from build123d import *

# Parameters (mm, degrees)
SKETCH1_W           = 50.8
SKETCH1_H           = 76.2
BOSS_EXTRUDE2_DEPTH = 20
SKETCH2_R           = 3.7
BOSS_EXTRUDE3_DEPTH = 2
CHAMFER7_SIZE       = 2.222212054
CHAMFER7_SIZE_2     = 25.4
FILLET6_R           = 2
FILLET7_R           = 2
FILLET8_R           = 2
FILLET9_R           = 2
FILLET10_R          = 2


with BuildPart() as part:
    # Sketch1 → Boss-Extrude2 (new body)
    with BuildSketch(Plane(origin=(0, 0, 0), x_dir=(1, 0, 0), z_dir=(0, 1, 0))):
        Rectangle(SKETCH1_W, SKETCH1_H)
    extrude(amount=BOSS_EXTRUDE2_DEPTH)

    # Sketch2 → Boss-Extrude3 (add)
    with BuildSketch(Plane(origin=(0, 0, -38.1), x_dir=(-1, 0, 0), z_dir=(0, 0, -1))):
        with Locations((-15.4, 10)):
            Circle(SKETCH2_R)
        with Locations((15.4, 10)):
            Circle(SKETCH2_R)
    extrude(amount=BOSS_EXTRUDE3_DEPTH)

    # Chamfer7
    # the kernel refuses this chamfer: 25.4, 2.222212054 mm, written as the material it takes off along each edge
    with BuildSketch(Plane(origin=(-25.4, -66.030705628, -38.1), x_dir=(-0.40120984275090654, 0, 0.9159861691531116), z_dir=(0, 1, 0))) as chamfer7_piece_1_section:
        Polygon((CHAMFER7_SIZE * 0.915986168971, CHAMFER7_SIZE * 0.401209842671), (-CHAMFER7_SIZE_2 * 0.401209842751, CHAMFER7_SIZE_2 * 0.915986169153), (0, 0), align=None)
    chamfer7_piece_1 = extrude(amount=152.061411256, mode=Mode.PRIVATE)
    chamfer7_piece_1 = chamfer7_piece_1 - Plane(origin=(-15.4, 10, -36.375506271), x_dir=(-1, 0, 0), z_dir=(0, 0, 1)) * Cylinder(3.7, 398, mode=Mode.PRIVATE)
    add(chamfer7_piece_1, mode=Mode.SUBTRACT)
    with BuildSketch(Plane(origin=(25.4, -66.030705628, -38.1), x_dir=(0.4012098427509076, 0, 0.9159861691531113), z_dir=(0, 1, 0))) as chamfer7_piece_2_section:
        Polygon((CHAMFER7_SIZE * 0.915986168971, -CHAMFER7_SIZE * 0.401209842671), (-CHAMFER7_SIZE_2 * 0.401209842751, -CHAMFER7_SIZE_2 * 0.915986169153), (0, 0), align=None)
    chamfer7_piece_2 = extrude(amount=152.061411256, mode=Mode.PRIVATE)
    chamfer7_piece_2 = chamfer7_piece_2 - Plane(origin=(15.4, 10, -36.375506337), x_dir=(-1, 0, 0), z_dir=(0, 0, 1)) * Cylinder(3.7, 398, mode=Mode.PRIVATE)
    add(chamfer7_piece_2, mode=Mode.SUBTRACT)

    # Fillet6
    fillet6_edges = [part.edges().sort_by_distance(p)[0] for p in [
        (25.4, 20, 1.111106027),
        (0, 20, 38.1),
        (12.7, 20, -36.988893973),
        (-12.7, 20, -36.988893973),
        (-25.4, 20, 1.111106027),
    ]]
    fillet(fillet6_edges, radius=FILLET6_R)

    # Fillet7
    # the kernel refuses this fillet: 2 mm, written as the material it takes off along each edge
    with BuildSketch(Plane(origin=(23.4, 18, -34.045125598), x_dir=(1, 0, 0), z_dir=(0, 1, 0))) as fillet7_piece_1_section:
        Polygon((0, 0), (FILLET7_R, 0), (FILLET7_R, FILLET7_R * 0.916331174017), (FILLET7_R * 0.0871557427476, FILLET7_R * 0.996194698092), align=None)
    fillet7_piece_1 = extrude(amount=FILLET7_R, mode=Mode.PRIVATE)
    fillet7_piece_1 = fillet7_piece_1 - Plane(origin=(23.4, 18, -34.045125598), x_dir=(-0.73727733681012, 0, 0.6755902076156647), z_dir=(0, 1, 0)) * Sphere(FILLET7_R, mode=Mode.PRIVATE)
    add(fillet7_piece_1, mode=Mode.SUBTRACT)
    with BuildSketch(Plane(origin=(25.4, -4.58165587, -35.877787946), x_dir=(0, 0, 1), z_dir=(0, 1, 0))) as fillet7_piece_2:
        with BuildLine():
            CenterArc((FILLET7_R * 0.916331174017, -FILLET7_R), FILLET7_R, 90, 85)
            Line((-FILLET7_R * 0.0798635240743, -FILLET7_R * 0.912844257252), (0, 0))
            Line((0, 0), (FILLET7_R * 0.916331174017, 0))
        make_face()
    extrude(amount=22.58165587, mode=Mode.SUBTRACT)

    # Fillet8
    # the kernel refuses this fillet: 2 mm, written as the material it takes off along each edge
    with BuildSketch(Plane(origin=(23.4, 18, 36.1), x_dir=(1, 0, 0), z_dir=(0, 0, 1))) as fillet8_piece_1_section:
        Polygon((0, 0), (FILLET8_R, 0), (FILLET8_R, FILLET8_R), (0, FILLET8_R), align=None)
    fillet8_piece_1 = extrude(amount=FILLET8_R, mode=Mode.PRIVATE)
    fillet8_piece_1 = fillet8_piece_1 - Plane(origin=(23.4, 18, 36.1), x_dir=(-0.7071067811865475, -0.7071067811865475, 0), z_dir=(0, 0, 1)) * Sphere(FILLET8_R, mode=Mode.PRIVATE)
    add(fillet8_piece_1, mode=Mode.SUBTRACT)
    with BuildSketch(Plane(origin=(25.4, -5, 38.1), x_dir=(-1, 0, 0), z_dir=(0, 1, 0))) as fillet8_piece_2:
        with BuildLine():
            CenterArc((FILLET8_R, -FILLET8_R), FILLET8_R, 90, 90)
            Line((0, -FILLET8_R), (0, 0))
            Line((0, 0), (FILLET8_R, 0))
        make_face()
    extrude(amount=23, mode=Mode.SUBTRACT)

    # Fillet9
    # the kernel refuses this fillet: 2 mm, written as the material it takes off along each edge
    with BuildSketch(Plane(origin=(-23.4, 18, 36.1), x_dir=(-1, 0, 0), z_dir=(0, 0, 1))) as fillet9_piece_1_section:
        Polygon((0, 0), (FILLET9_R, 0), (FILLET9_R, -FILLET9_R), (0, -FILLET9_R), align=None)
    fillet9_piece_1 = extrude(amount=FILLET9_R, mode=Mode.PRIVATE)
    fillet9_piece_1 = fillet9_piece_1 - Plane(origin=(-23.4, 18, 36.1), x_dir=(0.7071067811865475, -0.7071067811865475, 0), z_dir=(0, 0, 1)) * Sphere(FILLET9_R, mode=Mode.PRIVATE)
    add(fillet9_piece_1, mode=Mode.SUBTRACT)
    with BuildSketch(Plane(origin=(-25.4, -5, 38.1), x_dir=(1, 0, 0), z_dir=(0, 1, 0))) as fillet9_piece_2:
        with BuildLine():
            CenterArc((FILLET9_R, FILLET9_R), FILLET9_R, 180, 90)
            Line((0, FILLET9_R), (0, 0))
            Line((0, 0), (FILLET9_R, 0))
        make_face()
    extrude(amount=23, mode=Mode.SUBTRACT)

    # Fillet10
    # the kernel refuses this fillet: 2 mm, written as the material it takes off along each edge
    with BuildSketch(Plane(origin=(-23.4, 18, -34.045125598), x_dir=(-1, 0, 0), z_dir=(0, 1, 0))) as fillet10_piece_1_section:
        Polygon((0, 0), (FILLET10_R, 0), (FILLET10_R, -FILLET10_R * 0.916331174017), (FILLET10_R * 0.0871557427476, -FILLET10_R * 0.996194698092), align=None)
    fillet10_piece_1 = extrude(amount=FILLET10_R, mode=Mode.PRIVATE)
    fillet10_piece_1 = fillet10_piece_1 - Plane(origin=(-23.4, 18, -34.045125598), x_dir=(0.73727733681012, 0, 0.6755902076156647), z_dir=(0, 1, 0)) * Sphere(FILLET10_R, mode=Mode.PRIVATE)
    add(fillet10_piece_1, mode=Mode.SUBTRACT)
    with BuildSketch(Plane(origin=(-25.4, -4.58165587, -35.877787946), x_dir=(0, 0, 1), z_dir=(0, 1, 0))) as fillet10_piece_2:
        with BuildLine():
            CenterArc((FILLET10_R * 0.916331174017, FILLET10_R), FILLET10_R, 185, 85)
            Line((-FILLET10_R * 0.0798635240743, FILLET10_R * 0.912844257252), (0, 0))
            Line((0, 0), (FILLET10_R * 0.916331174017, 0))
        make_face()
    extrude(amount=22.58165587, mode=Mode.SUBTRACT)


solid = part.part
CAD build for the part. Positions are in the model's coordinates, mm. A direction names the side the tool comes from. Round coordinates to 2 decimals unless told otherwise and drop trailing zeros. Write each loop counter-clockwise with the first axis right and the second up, starting at its lowest first coordinate (ties: lowest second). Pieces come first, ordered by that corner, then holes. Notation, with made-up numbers: (25.25, 73) -> (30.25, 73) arc R16 ccw to (30.25, 103) -> close; hole circle Ø9 at (80, 42.5). An arc over 180 degrees is marked (long way). Answer as a JSON object with one key per item and string values.
(1) Band-saw the part on B-B, the plane y = 12. List the corners of the cut face in (x, z).
Reported:
{"outline": "(-25.4, -34.05) arc R2 ccw to (-23.57, -36.04) -> (-18.51, -36.48) -> (-18.51, -40.1) -> (-12.29, -40.1) -> (-12.29, -37.03) -> (0, -38.1) -> (12.29, -37.03) -> (12.29, -40.1) -> (18.51, -40.1) -> (18.51, -36.48) -> (23.57, -36.04) arc R2 ccw to (25.4, -34.05) -> (25.4, 36.1) arc R2 ccw to (23.4, 38.1) -> (-23.4, 38.1) arc R2 ccw to (-25.4, 36.1) -> close"}
(2) Band-saw the part on A-A, the plane y = 16.5. List the corners of the cut face in (x, z), then the cut area to 3 significant figures.
Reported:
{"outline": "(-25.4, -34.05) arc R2 ccw to (-23.57, -36.04) -> (0, -38.1) -> (23.57, -36.04) arc R2 ccw to (25.4, -34.05) -> (25.4, 36.1) arc R2 ccw to (23.4, 38.1) -> (-23.4, 38.1) arc R2 ccw to (-25.4, 36.1) -> close", "area": "3,810 mm^2"}
(3) Probe probe 1 along Z at (x, y) = (19, 13.25); probe 2 along Z at (x, y) = (20.5, 15). List the from-to ranges inside material, lowest first. Write a range as [from, to].
Reported:
{"probe 1": "z = [-36.44, 38.1]", "probe 2": "z = [-36.31, 38.1]"}
(4) Which spindle directions (+Z, -Z, +X, -X, +Y, -Y) get a long thin tool onto all of the face, cutting with end or side? Do faces 1 (the face through (-15, 10, -40.1)), 2 (the face through (-18.93, 8.89, -38.24)). Say none if no direction does.
Reported:
{"face 1": "-Z, +X, -X, +Y, -Y", "face 2": "-Z"}
(5) Two-plate mould, pull along X, no slides. Class faces 3 (the face through (-25.4, 9, 2)), 4 (the face through (15, 10, -40.1)), 5 (the face through (11.952, 6.874, -37.054)): +X half, -X half, draft (parallel to the pull), parting line (faces both ways), or undercut.
Reported:
{"face 3": "-X half", "face 4": "draft", "face 5": "undercut"}
(6) Pin check, flat tips, straight feed: P1, Ø1, axis at x = -17, y = 14, coming from the -Z side; P2, Ø4, axis at x = 0.5, y = 4, coming from the -Z side. Stop position of each tip, or through.
Reported:
{"P1": "stops at z = -36.66", "P2": "stops at z = -38.1"}
